The model under review builds one solid part; all positions refer to its coordinate system, in mm. A direction names the side the tool comes from. Round coordinates to 2 decimals unless told otherwise and drop trailing zeros. Order: outer loops, then holes, each group sorted by start corner. A loop starts at its lowest first (then second) coordinate and runs counter-clockwise, first axis right, second up. Notation, with made-up numbers: M 3,14 L 43,14 A9 cw 43,21 Z; hole C -16,29 d1. An arc over 180 degrees is marked long. Answer as a JSON object with one key per item and string values. Group by question number.
1) Consider section B-B, the plane z = -16.5. Write out the cut boundary in (x, y).
2) Consider section A-A, the plane x = -3. Write out the cut boundary in (y, z), then the cut area to 3 significant figures.
3) To check wall thickness, follow line 1 (X direction, y = 32, z = -6.25); line 2 (Z direction, x = -1.5, y = 33.5); line 3 (Y direction, x = -5, z = -0.75). State the ranges of each line that lie inside material, in increasing order.
4) Consider section D-D, the plane y = 41. Write out the cut boundary in (x, z), then the cut area to 3 significant figures.
5) Insertion check: pin 1 Ø6 at (x, z) = (-8, -5) entering from -Y; pin 2 Ø4 at (y, z) = (12.37, -8.43) entering from +X; pin 3 Ø1.5 at (x, y) = (-5.5, 16) entering from -Z. Each pin has a flat end and moves straight along its axis. Give the tip position at first contact, or say it passes through.
6) The part is to be moulded in two halves that separate along Y. For faces 3 (the flat face through (-4, 21, 0)), 4 (the cylindrical face through (0.199, 31.458, -8.707)), 5 (the flat face through (-9, -4.473, -10)), 6 (the cylindrical face through (-8.901, 31.458, -8.707)), say which applies: +Y half, -Y half, draft (parallel to the pull), parting line (faces both ways), or undercut.
7) Consider section C-C, the plane y = 5. Write out the cut boundary in (x, z), then the cut area to 3 significant figures.
8) For faces 1 (the cylindrical face through (-8.9, 10.31, -8.89)), 2 (the cylindrical face through (-0.53, 20.88, -1.2)), list the 3-axis set-ups (+Z, -Z, +X, -X, +Y, -Y) from which the entire face can be reached by the end or side of a thin tool; tool diameter is ignored.
```python
from build123d import *

# Parameters (mm, degrees)
SKETCH1_W                    = 8.2
SKETCH1_H                    = 50
BASE_FLANGE1_DEPTH           = 0.9
EDGE_FLANGE2_STRIP_W         = 5.6
EDGE_FLANGE2_STRIP_H         = 0.9
EDGE_FLANGE2_STRIP_CUT_DEPTH = 50
EDGE_FLANGE2_DEPTH           = 50
EDGE_FLANGE5_STRIP_W         = 5.6
EDGE_FLANGE5_STRIP_H         = 0.9
EDGE_FLANGE5_STRIP_CUT_DEPTH = 50
EDGE_FLANGE5_DEPTH           = 50
F_19_0_166_DIAMETER_SLOT1_D  = 4.2164
F_19_0_166_DIAMETER_SLOT2_D  = 4.2164


# Sheet-metal steps are written as plain solids
with BuildPart() as part:
    # Sketch1 → Base-Flange1 (new body)
    with BuildSketch(Plane.XY):
        with Locations((-4.344277108, 20.527108434)):
            Rectangle(SKETCH1_W, SKETCH1_H)
    extrude(amount=-BASE_FLANGE1_DEPTH)

    # Edge-Flange2 strip (across the edge) → Edge-Flange2 strip cut (cut)
    with BuildSketch(Plane(origin=(-8.444277108, -4.472891566, -0.9), x_dir=(1, 0, 0), z_dir=(0, 1, 0))):
        with Locations((-1.8, -0.45)):
            Rectangle(EDGE_FLANGE2_STRIP_W, EDGE_FLANGE2_STRIP_H)
    extrude(amount=EDGE_FLANGE2_STRIP_CUT_DEPTH, mode=Mode.SUBTRACT)

    # Edge-Flange2 section (across the edge) → Edge-Flange2 (add)
    with BuildSketch(Plane(origin=(-8.444277108, -4.472891566, -0.9), x_dir=(1, 0, 0), z_dir=(0, 1, 0))):
        with BuildLine():
            Line((-0.9, 1), (-0.9, 20))
            Line((-0.9, 20), (0, 20))
            Line((0, 20), (0, 1))
            ThreePointArc((0, 1), (0.292893219, 0.292893219), (1, 0))
            Line((1, 0), (1, -0.9))
            ThreePointArc((1, -0.9), (-0.343502884, -0.343502884), (-0.9, 1))
        make_face()
    extrude(amount=EDGE_FLANGE2_DEPTH)

    # Edge-Flange5 strip (across the edge) → Edge-Flange5 strip cut (cut)
    with BuildSketch(Plane(origin=(-0.244277108, 45.527108434, -0.9), x_dir=(-1, 0, 0), z_dir=(0, -1, 0))):
        with Locations((-1.8, -0.45)):
            Rectangle(EDGE_FLANGE5_STRIP_W, EDGE_FLANGE5_STRIP_H)
    extrude(amount=EDGE_FLANGE5_STRIP_CUT_DEPTH, mode=Mode.SUBTRACT)

    # Edge-Flange5 section (across the edge) → Edge-Flange5 (add)
    with BuildSketch(Plane(origin=(-0.244277108, 45.527108434, -0.9), x_dir=(-1, 0, 0), z_dir=(0, -1, 0))):
        with BuildLine():
            Line((-0.9, 1), (-0.9, 20))
            Line((-0.9, 20), (0, 20))
            Line((0, 20), (0, 1))
            ThreePointArc((0, 1), (0.292893219, 0.292893219), (1, 0))
            Line((1, 0), (1, -0.9))
            ThreePointArc((1, -0.9), (-0.343502884, -0.343502884), (-0.9, 1))
        make_face()
    extrude(amount=EDGE_FLANGE5_DEPTH)

    # #19 (0.166) Diameter Slot1 (through all)
    with Locations(Plane(origin=(0, 0, -0.9), x_dir=(-1, 0, 0), z_dir=(0, 0, -1))):
        with Locations((3.836019002, 40.527108434), (3.836019002, 0.527108434)):
            Hole(F_19_0_166_DIAMETER_SLOT1_D / 2)

    # #19 (0.166) Diameter Slot2 (through all)
    with Locations(Plane(origin=(0.655722892, 0, 0), x_dir=(0, 0, -1), z_dir=(1, 0, 0))):
        with Locations((8.432080696, 29.367284102), (8.432080696, 12.367284102)):
            Hole(F_19_0_166_DIAMETER_SLOT2_D / 2)


solid = part.part
```
Results list:
{
 "1": {"outline": "M -9.34,-4.47 L -8.44,-4.47 L -8.44,45.53 L -9.34,45.53 Z; M -0.24,-4.47 L 0.66,-4.47 L 0.66,45.53 L -0.24,45.53 Z"},
 "2": {"outline": "M -4.47,-0.9 L -1.41,-0.9 L -1.41,0 L -4.47,0 Z; M 2.46,-0.9 L 38.59,-0.9 L 38.59,0 L 2.46,0 Z; M 42.46,-0.9 L 45.53,-0.9 L 45.53,0 L 42.46,0 Z", "area": "38.0 mm^2"},
 "3": {"line 1": "-9.34 to -8.44, -0.24 to 0.66", "line 2": "-0.9 to 0", "line 3": "-4.47 to -1.23, 2.28 to 38.77, 42.28 to 45.53"},
 "4": {"outline": "M -9.34,-20.9 L -8.44,-20.9 L -8.44,-1.9 A1 cw -7.44,-0.9 L -5.89,-0.9 L -5.89,0 L -7.44,0 A1.9 ccw -9.34,-1.9 Z; M -1.78,-0.9 L -1.24,-0.9 A1 cw -0.24,-1.9 L -0.24,-20.9 L 0.66,-20.9 L 0.66,-1.9 A1.9 ccw -1.24,0 L -1.78,0 Z", "area": "40.2 mm^2"},
 "5": {"pin 1": "y = -4.47", "pin 2": "through", "pin 3": "z = -0.9"},
 "6": {"face 3": "draft", "face 4": "undercut", "face 5": "-Y half", "face 6": "undercut"},
 "7": {"outline": "M -9.34,-20.9 L -8.44,-20.9 L -8.44,-1.9 A1 cw -7.44,-0.9 L -1.24,-0.9 A1 cw -0.24,-1.9 L -0.24,-20.9 L 0.66,-20.9 L 0.66,-1.9 A1.9 ccw -1.24,0 L -7.44,0 A1.9 ccw -9.34,-1.9 Z", "area": "43.9 mm^2"},
 "8": {"face 1": "+X, -X", "face 2": "-Z, +Y, -Y"}
}
